Autodesk Inventor part; units mm, degrees
ref_plane "to_leaf2_XY" through (0, 1.9, 0) normal (0, 0, 1) x (1, 0, 0)
ref_plane "to_leaf2_YZ" through (0, 1.9, 0) normal (1, 0, 0) x (0, 1, 0)
ref_plane "to_leaf2_ZX" through (0, 1.9, 0) normal (0, 1, 0) x (0, 0, 1)
sketch "Sketch_15" plane through (0, 0, 0) normal (0, 0, 1) x (1, 0, 0)
  arc A0 (1.5492, 0.8) -> (0, 0) centre (0, 1.9) ccw
  line L0 (0, 0) -> (10, 0)
  line L1 (10, 0) -> (10, 0.8)
  line L2 (10, 0.8) -> (1.5492, 0.8)
  circle A1 centre (0, 1.9) radius 1
extrude "Extrusion1" add sketch "Sketch_15" against normal blind 25
sketch "Sketch_1" plane through (0, 0, 0) normal (0, 1, 0) x (-1, 0, 0)
  line L0 (6, -25) -> (6, 0)
  line L1 (6, 0) -> (-2.09, 0)
  line L2 (-2.09, 0) -> (-2.09, -8.3333)
  line L3 (-2.09, -8.3333) -> (2.09, -8.3333)
  line L4 (2.09, -8.3333) -> (2.09, -16.6667)
  line L5 (2.09, -16.6667) -> (-2.09, -16.6667)
  line L6 (-2.09, -16.6667) -> (-2.09, -25)
  line L7 (-2.09, -25) -> (6, -25)
extrude "Extrusion2" cut sketch "Sketch_1" along normal blind 3.8
sketch "Sketch3" plane through (10, 0, -25) normal (0, -1, 0) x (1, 0, 0)
  point P0 (-4, 4.5)
hole "Hole1" at (6, 0, -20.5) direction (0, 1, 0) diameter 3.4 depth 0.8
pattern_linear "Rectangular Pattern1" count 2 spacing 16 along (0, 0, 1) of "Hole1"
ref_plane "to_leaf2_XY" through (0, 1.9, 0) normal (0, 0, 1) x (1, 0, 0)
ref_plane "to_leaf2_YZ" through (0, 1.9, 0) normal (1, 0, 0) x (0, 1, 0)
ref_plane "to_leaf2_ZX" through (0, 1.9, 0) normal (0, 1, 0) x (0, 0, 1)
properties part number "HHS25-LEAF1"
Work out the finished part from the listing and answer in its coordinate system (mm). A direction names the side the tool comes from. Give positions to 0.01 mm unless a question says otherwise; leave off trailing zeros. Loops run counter-clockwise (first coordinate to the right, second up) from the corner with the lowest first, then second, coordinate; pieces in that order, holes last. Notation, with made-up numbers: (75.5, -30) -> (116.5, -30) arc R14 cw to (116.5, -20) -> close; hole circle Ø5 at (66, 48). An arc over 180 degrees is marked (long way). Use a Markdown table: item, result. Add a question column.
1. Section C-C on z = -20.5 is taken. Determine the outline of the cut face in (x, y).
2. Determine the mould class of faces 3 (the cylindrical face through (7.5, 0.4, -5.3)), 4 (the flat face through (1, 1, -8.333)) for opening direction X: released by +X, released by -X, zero draft, split by the parting line, or undercut.
3. For faces 1 (the flat face through (1, 1, -16.667)), 2 (the cylindrical face through (-0.217, 0.924, -12.442)), determine the directions among +Z, -Z, +X, -X, +Y, -Y from which every point of the face is accessible in a straight line to the end or side of a thin tool.
4. Section B-B on y = 1.9 is taken. Determine the outline of the cut face in (x, z).
5. Find the intervals of material crossed by probe 1 along Z at (x, y) = (6, 0.4); probe 2 along Y at (x, z) = (0, -13.5); probe 3 along X at (y, z) = (0.35, -4.5), in increasing order.
6. Section A-A on x = 6 is taken. Determine the outline of the cut face in (y, z), and give its area (3 significant figures).
7. Section D-D on y = 0.4 is taken. Determine the outline of the cut face in (x, z).
8. A flat-ended cylindrical pin translates along its axis: pin 1 Ø2.5 at (x, z) = (4, -13.5) entering from +Y. Find the tip coordinate at first contact, or state that the pin passes through.
Results below:
| question | item | result |
|---|---|---|
| 1 | outline | (2.09, 0) -> (4.3, 0) -> (4.3, 0.8) -> (2.09, 0.8) -> close; (7.7, 0) -> (10, 0) -> (10, 0.8) -> (7.7, 0.8) -> close |
| 2 | face 3 | undercut |
| 2 | face 4 | zero draft |
| 3 | face 1 | -Z, -X, +Y, -Y |
| 3 | face 2 | +Z, -Z |
| 4 | outline | (-1.9, -16.67) -> (-1, -16.67) -> (-1, -8.33) -> (-1.9, -8.33) -> close; (1, -16.67) -> (1.9, -16.67) -> (1.9, -8.33) -> (1, -8.33) -> close |
| 5 | probe 1 | z = -25 to -22.2, -18.8 to -6.2, -2.8 to 0 |
| 5 | probe 2 | y = 0 to 0.9, 2.9 to 3.8 |
| 5 | probe 3 | x = 2.09 to 4.3, 7.7 to 10 |
| 6 | outline | (0, -25) -> (0.8, -25) -> (0.8, -22.2) -> (0, -22.2) -> close; (0, -18.8) -> (0.8, -18.8) -> (0.8, -6.2) -> (0, -6.2) -> close; (0, -2.8) -> (0.8, -2.8) -> (0.8, 0) -> (0, 0) -> close |
| 6 | area | 14.6 mm^2 |
| 7 | outline | (-1.17, -16.67) -> (2.09, -16.67) -> (2.09, -25) -> (10, -25) -> (10, 0) -> (2.09, 0) -> (2.09, -8.33) -> (-1.17, -8.33) -> close; hole circle Ø3.4 at (6, -20.5); hole circle Ø3.4 at (6, -4.5) |
| 8 | pin 1 | stops at y = 0.8 |
